The model under review builds one solid part; all positions refer to its coordinate system, in mm. A direction names the side the tool comes from. Coordinates: 2 decimals unless noted, no trailing zeros. Loops run counter-clockwise (first coordinate to the right, second up) from the corner with the lowest first, then second, coordinate; pieces in that order, holes last. Notation, with made-up numbers: M 72,72.25 L 82,72.25 A29 cw 82,105.25 Z; hole C 46.5,82.5 d6. An arc over 180 degrees is marked long. Return JSON: item names as keys, results as strings.
```python
from build123d import *

# Parameters (mm, degrees)
F0_W     = 35.56
F0_H     = 15.24
F1_DEPTH = 17.78
F2_R     = 2.54
F3_DEPTH = 25.4
F4_R     = 2.54
F5_DEPTH = 25.4


with BuildPart() as f1:
    # F0 (on Front) → F1 (new body)
    with BuildSketch(Plane.XZ):
        with Locations((-1.695781, 7.62)):
            Rectangle(F0_W, F0_H)
    extrude(amount=F1_DEPTH)

    # F2 (on Right) → F3 (cut)
    with BuildSketch(Plane.YZ):
        with Locations((-8.775705, 0)):
            Circle(F2_R)
    extrude(amount=F3_DEPTH, mode=Mode.SUBTRACT)

    # F4 (on Right) → F5 (cut)
    with BuildSketch(Plane.YZ):
        with Locations((-8.858354, 0)):
            Circle(F4_R)
    extrude(amount=-F5_DEPTH, mode=Mode.SUBTRACT)


solid = f1.part
```
1. The part is to be moulded in two halves that separate along Y. For faces 3 (the face through (16.084, -9, 8)), 4 (the face through (-2, -17.78, 8)), 5 (the face through (-9.6, -8.8, 2.54)), say which applies: released by +Y, released by -Y, zero draft, split by the parting line, or undercut.
Check values:
{"face 3": "zero draft", "face 4": "released by -Y", "face 5": "undercut"}
2. Add section B-B on y = -6.75. Give the boundary of the cut face in (x, z), plus the area to 3 significant figures.
Check values:
{"outline": "M -19.48,1.42 L 0,1.42 L 0,1.53 L 16.08,1.53 L 16.08,15.24 L -19.48,15.24 Z", "area": "490 mm²"}
3. Machinability: for faces 1 (the face through (-2, -9, 15.24)), 2 (the face through (7.93, -8.72, 2.54)), which of the approach directions +Z, -Z, +X, -X, +Y, -Y give a long, thin tool a straight path to every point of the face, cutting with its end or side? Answer none if there is none.
Check values:
{"face 1": "+Z, +X, -X, +Y, -Y", "face 2": "-Z, +X"}
4. Add section A-A on x = -7. Give the boundary of the cut face in (y, z), plus the area to 3 significant figures.
Check values:
{"outline": "M -17.78,0 L -11.4,0 A2.54 cw -6.32,0 L 0,0 L 0,15.24 L -17.78,15.24 Z", "area": "261 mm²"}
5. To check wall thickness, follow line 1 (Y direction, x = -10.5, z = 1); line 2 (Y direction, x = 8.5, z = 0.5); line 3 (Z direction, x = -0.5, y = -7.75). State the ranges of each line that lie inside material, in increasing order.
Check values:
{"line 1": "-17.78 to -11.19, -6.52 to 0", "line 2": "-17.78 to -11.27, -6.29 to 0", "line 3": "2.29 to 15.24"}
6. Insertion check: pin 1 Ø0.8 at (y, z) = (-9.5, 0.5) entering from -X. The pin has a flat end and moves straight along its axis. Give the tip position at first contact, or say it passes through.
Check values:
{"pin 1": "through"}
